from build123d import *

# Parameters (mm, degrees)
F1_DEPTH = 26.9878935069
F2_R     = 10.5222192306
F3_DEPTH = 26.9888935069
F4_SIZE  = 2.54
F5_SIZE  = 2.54


with BuildPart() as f1:
    # F0 (on Front) → F1 (new body)
    with BuildSketch(Plane.XZ):
        Polygon((26.283480227, -21.57907933), (26.283480227, 21.4828625321), (-18.810749054, 21.2165787816), (-18.810749054, -21.57907933), align=None)
    extrude(amount=-F1_DEPTH)

    # F2 (on face) → F3 (cut, through all)
    with BuildSketch(Plane.XZ):
        Circle(F2_R)
    extrude(amount=-F3_DEPTH, mode=Mode.SUBTRACT)

    # F4
    f4_edges = [f1.edges().sort_by_distance(p)[0] for p in [
        (26.28348, 26.987894, -0.048108),
        (3.736366, 26.987894, -21.579079),
        (3.736366, 26.987894, 21.349721),
        (-18.810749, 26.987894, -0.18125),
        (-10.522219, 26.987894, 0),
    ]]
    chamfer(f4_edges, length=F4_SIZE)

    # F5
    f5_edges = [f1.edges().sort_by_distance(p)[0] for p in [
        (26.28348, 0, -0.048108),
        (3.736366, 0, -21.579079),
        (3.736366, 0, 21.349721),
        (-18.810749, 0, -0.18125),
        (-10.522219, 0, 0),
    ]]
    chamfer(f5_edges, length=F5_SIZE)


solid = f1.part
Input: part model. Units: mm. Frame: model coordinates. Coordinates: 2 decimals unless noted, no trailing zeros. Loops run counter-clockwise (first coordinate to the right, second up) from the corner with the lowest first, then second, coordinate; pieces in that order, holes last.
Q1. Cut plane A-A (z = 0). Output: boundary loops of the cut face in (x, y).
Q2. Material intervals for line 1 (X direction, y = 1.75, z = 8); line 2 (Z direction, x = 0, y = 8); line 3 (Z direction, x = -5, y = 15), sorted ascending.
Q3. Cut plane B-B (y = 13.75). Output: boundary loops of the cut face in (x, z).
Q4. Cut plane C-C (x = -14). Output: boundary loops of the cut face in (y, z), then the cut area to 3 significant figures.
Q5. Contact query for flat-ended pins moving along their axis: pin 1 (8 mm diameter, centred on x = -6, y = 4.5, fed in from +Z); pin 2 (12 mm diameter, centred on x = 14, y = 8, fed in from +Z). Output: stop coordinate, or through.
Q6. Draft query along X for faces 1 (the face through (12, 26.988, 9)), 2 (the face through (-8.448, 24.571, -6.478)), 3 (the face through (-17.56, 25.7, 0.12)). Return one class per face: +X half, -X half, draft (parallel to the pull), parting line (faces both ways), or undercut.
Working result:
1. outline: (-18.81, 2.54) - (-16.27, 0) - (-13.06, 0) - (-10.52, 2.54) - (-10.52, 24.45) - (-13.06, 26.99) - (-16.27, 26.99) - (-18.81, 24.45) - close; (10.52, 2.54) - (13.06, 0) - (23.74, 0) - (26.28, 2.54) - (26.28, 24.45) - (23.74, 26.99) - (13.06, 26.99) - (10.52, 24.45) - close
2. line 1: x = -18.02 to -8, 8 to 25.49
2. line 2: z = -21.58 to -10.52, 10.52 to 21.33
2. line 3: z = -21.58 to -9.26, 9.26 to 21.3
3. outline: (-18.81, -21.58) - (26.28, -21.58) - (26.28, 21.48) - (-18.81, 21.22) - close; hole circle Ø21.04 at (0, 0)
4. outline: (0, -19.04) - (2.54, -21.58) - (24.45, -21.58) - (26.99, -19.04) - (26.99, 18.7) - (24.45, 21.24) - (2.54, 21.24) - (0, 18.7) - close
4. area: 1,140 mm2
5. pin 1: stops at z = 21.32
5. pin 2: stops at z = 21.45
6. face 1: draft
6. face 2: undercut
6. face 3: -X half
